Input: part model. Units: mm. Frame: model coordinates. A direction names the side the tool comes from. Round coordinates to 2 decimals unless told otherwise and drop trailing zeros. Write each loop counter-clockwise with the first axis right and the second up, starting at its lowest first coordinate (ties: lowest second). Pieces come first, ordered by that corner, then holes. Notation, with made-up numbers: (-24, 19) -> (4, 19) arc R26 cw to (4, 57) -> close; hole circle Ø5 at (-7, -39.75). An arc over 180 degrees is marked (long way). Write item = value, one per line.
```python
from build123d import *

# Parameters (mm, degrees)
BOSS_EXTRU_1_DEPTH      = 2
ESQUISSE2_W             = 2
ESQUISSE2_H             = 43.4
BOSS_EXTRU_2_DEPTH      = 23
ESQUISSE3_W             = 2
ESQUISSE3_H             = 23
BOSS_EXTRU_3_DEPTH      = 8
ESQUISSE8_W             = 2
ESQUISSE8_H             = 23
BOSS_EXTRU_5_DEPTH      = 8
ESQUISSE9_R             = 2
ENL_V_MAT_EXTRU_3_DEPTH = 2
ESQUISSE10_R            = 1.5
ENL_V_MAT_EXTRU_4_DEPTH = 2


with BuildPart() as part:
    # Esquisse1 → Boss.-Extru.1 (new body)
    with BuildSketch(Plane.XY):
        Polygon((8.75, 17), (8.75, 19), (13.75, 19), (13.75, 27), (-10.25, 27), (-10.25, 19), (-18.25, 19), (-18.25, -24.4), (-10.25, -24.4), (-10.25, -32.4), (13.75, -32.4), (13.75, -24.4), (8.75, -24.4), (8.75, -22.4), (18.25, -22.4), (18.25, 17), align=None)
    extrude(amount=BOSS_EXTRU_1_DEPTH)

    # Esquisse2 → Boss.-Extru.2 (add)
    with BuildSketch(Plane(origin=(0, 0, 0), x_dir=(-1, 0, 0), z_dir=(0, 0, -1))):
        with Locations((17.25, -2.7)):
            Rectangle(ESQUISSE2_W, ESQUISSE2_H)
    extrude(amount=BOSS_EXTRU_2_DEPTH)

    # Esquisse3 → Boss.-Extru.3 (add)
    with BuildSketch(Plane(origin=(0, 27, 0), x_dir=(1, 0, 0), z_dir=(0, 1, 0))):
        with Locations((12.75, 11.5)):
            Rectangle(ESQUISSE3_W, ESQUISSE3_H)
    extrude(amount=-BOSS_EXTRU_3_DEPTH)

    # Esquisse8 → Boss.-Extru.5 (add)
    with BuildSketch(Plane.XZ.offset(32.4)):
        with Locations((12.75, -11.5)):
            Rectangle(ESQUISSE8_W, ESQUISSE8_H)
    extrude(amount=-BOSS_EXTRU_5_DEPTH)

    # Esquisse9 → Enlèv. mat.-Extru.3 (cut)
    with BuildSketch(Plane(origin=(13.75, 0, 0), x_dir=(0, 0, -1), z_dir=(1, 0, 0))):
        with Locations((5.2, 22.5)):
            Circle(ESQUISSE9_R)
        with Locations((15.2, 22.5)):
            Circle(ESQUISSE9_R)
        with Locations((15.2, -27.9)):
            Circle(ESQUISSE9_R)
        with Locations((5.2, -27.9)):
            Circle(ESQUISSE9_R)
    extrude(amount=-ENL_V_MAT_EXTRU_3_DEPTH, mode=Mode.SUBTRACT)

    # Esquisse10 → Enlèv. mat.-Extru.4 (cut)
    with BuildSketch(Plane.ZY.offset(18.25)):
        with Locations((-11, 15.5)):
            Circle(ESQUISSE10_R)
        with Locations((-11, 8.5)):
            Circle(ESQUISSE10_R)
        with Locations((-4, 8.5)):
            Circle(ESQUISSE10_R)
        with Locations((-11, 1.5)):
            Circle(ESQUISSE10_R)
        with Locations((-18, 8.5)):
            Circle(ESQUISSE10_R)
        with Locations((-11, -6.9)):
            Circle(ESQUISSE10_R)
        with Locations((-11, -13.9)):
            Circle(ESQUISSE10_R)
        with Locations((-4, -13.9)):
            Circle(ESQUISSE10_R)
        with Locations((-18, -13.9)):
            Circle(ESQUISSE10_R)
        with Locations((-11, -20.9)):
            Circle(ESQUISSE10_R)
    extrude(amount=-ENL_V_MAT_EXTRU_4_DEPTH, mode=Mode.SUBTRACT)


solid = part.part
```
1) Line query: L1, parallel to Y at x = 13.1, z = -15.2; L2, parallel to Y at x = -16.85, z = -18; L3, parallel to X at y = -13.5, z = -21.75. Output: solid intervals per line, ascending. Write a range as from..to.
Solutions:
L1 = -32.4..-29.9, -25.9..-24.4, 19..20.5, 24.5..27
L2 = -24.4..-15.4, -12.4..7, 10..19
L3 = -18.25..-16.25
2) Cut plane D-D (y = 8.5). Return the cut outline in (x, z), and give its area (3 significant figures).
Solutions:
outline = (-18.25, -23) -> (-16.25, -23) -> (-16.25, -19.5) -> (-18.25, -19.5) -> close; (-18.25, -16.5) -> (-16.25, -16.5) -> (-16.25, -12.5) -> (-18.25, -12.5) -> close; (-18.25, -9.5) -> (-16.25, -9.5) -> (-16.25, -5.5) -> (-18.25, -5.5) -> close; (-18.25, -2.5) -> (-16.25, -2.5) -> (-16.25, 0) -> (18.25, 0) -> (18.25, 2) -> (-18.25, 2) -> close
area = 101 mm^2
3) Cut plane C-C (z = -15.2). Return the cut outline in (x, y), and give its area (3 significant figures).
Solutions:
outline = (-18.25, -24.4) -> (-16.25, -24.4) -> (-16.25, 19) -> (-18.25, 19) -> close; (11.75, -32.4) -> (13.75, -32.4) -> (13.75, -29.9) -> (11.75, -29.9) -> close; (11.75, -25.9) -> (13.75, -25.9) -> (13.75, -24.4) -> (11.75, -24.4) -> close; (11.75, 19) -> (13.75, 19) -> (13.75, 20.5) -> (11.75, 20.5) -> close; (11.75, 24.5) -> (13.75, 24.5) -> (13.75, 27) -> (11.75, 27) -> close
area = 103 mm^2
4) First-contact query: P1, Ø4, axis at y = 24, z = -14, coming from the +X side; P2, Ø3.5, axis at y = -13.9, z = -18, coming from the -X side; P3, Ø1.6, axis at y = 24.5, z = 1, coming from the -X side; P4, Ø11.5, axis at y = -7.5, z = -13.5, coming from the +X side. Flat tips, straight axial feed; report the tip coordinate or a pass-through.
Solutions:
P1 = 13.75
P2 = -18.25
P3 = -10.25
P4 = -16.25
5) Draft query along Z for faces 1 (the face through (-17.3, 7.6, -12.2)), 2 (the face through (11.75, 23, -11)). Return one class per face: +Z half, -Z half, draft (parallel to the pull), parting line (faces both ways), or undercut.
Solutions:
face_1 = undercut
face_2 = draft
6) Cut plane B-B (y = 15.5). Return the cut outline in (x, z).
Solutions:
outline = (-18.25, -23) -> (-16.25, -23) -> (-16.25, -12.5) -> (-18.25, -12.5) -> close; (-18.25, -9.5) -> (-16.25, -9.5) -> (-16.25, 0) -> (18.25, 0) -> (18.25, 2) -> (-18.25, 2) -> close
7) Cut plane A-A (x = 13). Return the cut outline in (y, z).
Solutions:
outline = (-32.4, -23) -> (-24.4, -23) -> (-24.4, 2) -> (-32.4, 2) -> close; (-22.4, 0) -> (17, 0) -> (17, 2) -> (-22.4, 2) -> close; (19, -23) -> (27, -23) -> (27, 2) -> (19, 2) -> close; hole circle Ø4 at (-27.9, -15.2); hole circle Ø4 at (-27.9, -5.2); hole circle Ø4 at (22.5, -15.2); hole circle Ø4 at (22.5, -5.2)
8) Access query for faces 3 (the face through (-17, 19, -8)), 4 (the face through (-17, 7, -4)), 5 (the face through (14, 17, 1)), 6 (the face through (12, -32.4, -5)), 7 (the face through (-17, -24.4, -8)). Directions: +Z, -Z, +X, -X, +Y, -Y. A direction counts if a zero-diameter tool reaches every point of the face in a straight line with its end or side. Return the directions, or none.
Solutions:
face_3 = +Z, -Z, -X, +Y
face_4 = +X, -X
face_5 = +Z, -Z, +X
face_6 = +Z, -Z, +X, -X, -Y
face_7 = +Z, -Z, -X, -Y
